Could you check a few things on this drawing? It's one solid part, dimensions in mm from its lowest x, y, z. Give positions to 0.01 mm unless a question says otherwise; leave off trailing zeros. Order: outer loops, then holes, each group sorted by start corner. A loop starts at its lowest first (then second) coordinate and runs counter-clockwise, first axis right, second up. Notation, with made-up numbers: M -20,-24.5 L 33,-24.5 A30 cw 33,7.5 Z; hole C -38,85.5 d3. An arc over 180 degrees is marked long. Use one line per item in the form item = value. Start each with the question number.
1. I want a section at C-C, the plane z = 2. List the corners of the cut face in (x, y) for me (1 decimal).
2. I want a section at B-B, the plane x = 13.5. List the corners of the cut face in (y, z) for me (1 decimal).
3. I need wall thicknesses on L1, parallel to Z at x = 19.5, y = 2.5 (1 decimal); L2, parallel to X at y = 7.25, z = 4.75 (1 decimal); L3, parallel to X at y = 5, z = 7 (1 decimal). Which ranges of each line are inside material? Lowest first, please.
4. I want a section at D-D, the plane y = 3. List the corners of the cut face in (x, z) for me (1 decimal).
5. I want a section at A-A, the plane y = 7.25. List the corners of the cut face in (x, z) for me (1 decimal).
6. We'd pull the mould along Z, two halves only. Please class the marked faces 1, 2, 3 and 4: +Z half, -Z half, draft (parallel to the pull), parting line (faces both ways), or undercut.
7. Will these pins go through, and if not, where does the flat tip stop? P1, Ø4, axis at y = 2, z = 1.5, coming from the +X side; P2, Ø1.5, axis at y = 7.5, z = 6.5, coming from the +X side; P3, Ø1, axis at x = 8.5, z = 8.5, coming from the +Y side.
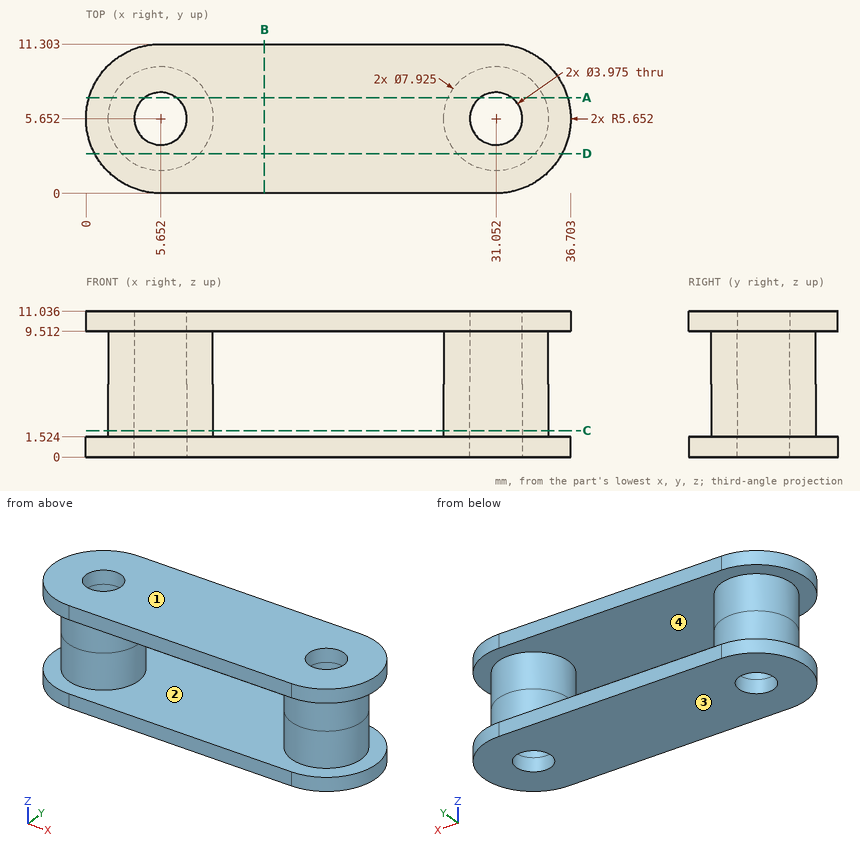
Check result:
q1.outline = C 5.7,5.7 d7.9; C 31.1,5.7 d7.9; hole C 5.7,5.7 d4; hole C 31.1,5.7 d4
q2.outline = M 0,0 L 11.3,0 L 11.3,1.5 L 0,1.5 Z; M 0,9.5 L 11.3,9.5 L 11.3,11 L 0,11 Z
q3.L1 = 0 to 1.5, 9.5 to 11
q3.L2 = 2 to 4.5, 6.8 to 9.3, 27.4 to 29.9, 32.2 to 34.7
q3.L3 = 1.7 to 3.8, 7.5 to 9.6, 27.1 to 29.2, 32.9 to 35
q4.outline = M 0.7,0 L 36,0 L 36,1.5 L 34,1.5 L 34,9.5 L 36,9.5 L 36,11 L 0.7,11 L 0.7,9.5 L 2.7,9.5 L 2.7,1.5 L 0.7,1.5 Z; hole M 8.6,1.5 L 28.1,1.5 L 28.1,9.5 L 8.6,9.5 Z
q5.outline = M 0.2,0 L 4.5,0 L 4.5,11 L 0.2,11 L 0.2,9.5 L 2,9.5 L 2,1.5 L 0.2,1.5 Z; M 6.8,0 L 29.9,0 L 29.9,11 L 6.8,11 Z; M 32.2,0 L 36.5,0 L 36.5,1.5 L 34.7,1.5 L 34.7,9.5 L 36.5,9.5 L 36.5,11 L 32.2,11 Z; hole M 9.3,1.5 L 27.4,1.5 L 27.4,9.5 L 9.3,9.5 Z
q6.face_1 = +Z half
q6.face_2 = undercut
q6.face_3 = -Z half
q6.face_4 = undercut
q7.P1 = 36.46
q7.P2 = 34.86
q7.P3 = 8.84
